from build123d import *

# Parameters (mm, degrees)
SKETCH3_W           = 22.2
SKETCH3_H           = 42.9
BOSS_EXTRUDE2_DEPTH = 20
SKETCH4_R           = 8
CUT_EXTRUDE1_DEPTH  = 5
SKETCH5_R           = 8
CUT_EXTRUDE2_DEPTH  = 5
SKETCH11_R          = 10
BOSS_EXTRUDE3_DEPTH = 39.2
SKETCH13_R          = 10
SKETCH13_R_2        = 7
CUT_EXTRUDE5_DEPTH  = 23.52
SKETCH14_R          = 7
SKETCH14_R_2        = 5.5
CUT_EXTRUDE6_DEPTH  = 7.84
CHAMFER2_SIZE       = 1
SKETCH15_R          = 5.5
SKETCH15_R_2        = 4
CUT_EXTRUDE7_DEPTH  = 3
SKETCH16_R          = 10
BOSS_EXTRUDE4_DEPTH = 10


with BuildPart() as part:
    # Sketch3 → Boss-Extrude2 (new body)
    with BuildSketch(Plane(origin=(0, 0, 0), x_dir=(0, 0, -1), z_dir=(1, 0, 0))):
        Rectangle(SKETCH3_W, SKETCH3_H)
    extrude(amount=BOSS_EXTRUDE2_DEPTH)

    # Sketch4 → Cut-Extrude1 (cut)
    with BuildSketch(Plane(origin=(0, 21.45, 0), x_dir=(1, 0, 0), z_dir=(0, 1, 0))):
        with Locations((10, 0)):
            Circle(SKETCH4_R)
    extrude(amount=-CUT_EXTRUDE1_DEPTH, mode=Mode.SUBTRACT)

    # Sketch5 → Cut-Extrude2 (cut)
    with BuildSketch(Plane.XZ.offset(21.45)):
        with Locations((10, 0)):
            Circle(SKETCH5_R)
    extrude(amount=-CUT_EXTRUDE2_DEPTH, mode=Mode.SUBTRACT)

    # Sketch11 → Boss-Extrude3 (add)
    with BuildSketch(Plane(origin=(0, 0, -11.1), x_dir=(-1, 0, 0), z_dir=(0, 0, -1))):
        with Locations((-10, 0)):
            Circle(SKETCH11_R)
    extrude(amount=BOSS_EXTRUDE3_DEPTH)

    # Sketch13 → Cut-Extrude5 (cut)
    with BuildSketch(Plane(origin=(0, 0, -50.3), x_dir=(-1, 0, 0), z_dir=(0, 0, -1))):
        with Locations((-10, 0)):
            Circle(SKETCH13_R)
        with Locations((-10, 0)):
            Circle(SKETCH13_R_2, mode=Mode.SUBTRACT)
    extrude(amount=-CUT_EXTRUDE5_DEPTH, mode=Mode.SUBTRACT)

    # Sketch14 → Cut-Extrude6 (cut)
    with BuildSketch(Plane(origin=(0, 0, -50.3), x_dir=(-1, 0, 0), z_dir=(0, 0, -1))):
        with Locations((-10, 0)):
            Circle(SKETCH14_R)
        with Locations((-10, 0)):
            Circle(SKETCH14_R_2, mode=Mode.SUBTRACT)
    extrude(amount=-CUT_EXTRUDE6_DEPTH, mode=Mode.SUBTRACT)

    # Chamfer2
    chamfer2_edges = [part.edges().sort_by_distance(p)[0] for p in [
        (15.5, 0, -50.3),
    ]]
    chamfer(chamfer2_edges, length=CHAMFER2_SIZE)

    # Sketch15 → Cut-Extrude7 (cut)
    with BuildSketch(Plane(origin=(0, 0, -42.46), x_dir=(-1, 0, 0), z_dir=(0, 0, -1))):
        with Locations((-10, 0)):
            Circle(SKETCH15_R)
        with Locations((-10, 0)):
            Circle(SKETCH15_R_2, mode=Mode.SUBTRACT)
    extrude(amount=CUT_EXTRUDE7_DEPTH, mode=Mode.SUBTRACT)

    # Sketch16 → Boss-Extrude4 (add)
    with BuildSketch(Plane.XY.offset(11.1)):
        with Locations((10, 0)):
            Circle(SKETCH16_R)
    extrude(amount=BOSS_EXTRUDE4_DEPTH)


solid = part.part
Verification items for the finished model (mm, model axes). A direction names the side the tool comes from. Round coordinates to 2 decimals unless told otherwise and drop trailing zeros. Loops run counter-clockwise (first coordinate to the right, second up) from the corner with the lowest first, then second, coordinate; pieces in that order, holes last. Notation, with made-up numbers: (69, -22.5) - (107, -22.5) arc R12 ccw to (107, -18.5) - close; hole circle Ø2 at (3.5, -16.75). An arc over 180 degrees is marked (long way). Use a Markdown table: item, result. Add a question column.
1. Section check B-B, the plane z = 0. Record the boundary of the cut face in (x, y).
2. Release check for a two-part mould opening along X. For faces 1 (the face through (8.27, 18.98, 7.81)), 2 (the face through (4.92, -2.11, -47.41)), 3 (the face through (3, 21.45, -5)) record: released by +X, released by -X, zero draft, split by the parting line, or undercut.
3. Gauge pin test, flat ends, axial feed: pin 1 (6 mm diameter, centred on x = 6, y = 14, fed in from -Z); pin 2 (1.5 mm diameter, centred on x = 13.5, z = -4, fed in from -Y); pin 3 (8 mm diameter, centred on y = -8.5, z = -27, fed in from -X). Record the tip position at first contact, or that the pin passes through.
4. Thickness scan on probe 1 along Z at (x, y) = (10, 17.5); probe 2 along X at (y, z) = (19.8, 0); probe 3 along Z at (x, y) = (5, 8). Record the ranges inside material, lowest first. Write a range as [from, to].
5. Section check A-A, the plane y = 19.5. Record the boundary of the cut face in (x, z), plus the area to 3 significant figures.
6. Access from +Z, -Z, +X, -X, +Y, -Y to the whole of each face (thin tool, end or side, straight path). Record for faces 4 (the face through (3, -21.45, -5)), 5 (the face through (17, -2, -26.78)), 6 (the face through (10, -16.45, 0)), 7 (the face through (0, 0, 16)), 8 (the face through (13.2, -2.4, -43.9)).
7. Section check D-D, the plane y = -15.5. Record the boundary of the cut face in (x, z), plus the area to 3 significant figures.
Checks:
| question | item | result |
|---|---|---|
| 1 | outline | (0, -21.45) - (2, -21.45) - (2, -16.45) - (18, -16.45) - (18, -21.45) - (20, -21.45) - (20, 21.45) - (18, 21.45) - (18, 16.45) - (2, 16.45) - (2, 21.45) - (0, 21.45) - close |
| 2 | face 1 | undercut |
| 2 | face 2 | split by the parting line |
| 2 | face 3 | zero draft |
| 3 | pin 1 | stops at z = -11.1 |
| 3 | pin 2 | stops at y = -16.45 |
| 3 | pin 3 | stops at x = 1.07 |
| 4 | probe 1 | z = [-11.1, -8], [8, 11.1] |
| 4 | probe 2 | x = [0, 2], [18, 20] |
| 4 | probe 3 | z = [-26.78, 21.1] |
| 5 | outline | (0, -11.1) - (20, -11.1) - (20, 11.1) - (0, 11.1) - close; hole circle Ø16 at (10, 0) |
| 5 | area | 243 mm^2 |
| 6 | face 4 | +Z, -Z, +X, -X, -Y |
| 6 | face 5 | -Z |
| 6 | face 6 | -Y |
| 6 | face 7 | +Z |
| 6 | face 8 | none |
| 7 | outline | (0, -11.1) - (20, -11.1) - (20, 11.1) - (0, 11.1) - close |
| 7 | area | 444 mm^2 |
